```python
from build123d import *

# Parameters (mm, degrees)
F0_R     = 24.686614
F1_DEPTH = 127
F2_R     = 5.08
F3_W     = 13.125889
F3_H     = 11.96772
F4_DEPTH = 127.001


with BuildPart() as f1:
    # F0 (on Front) → F1 (new body)
    with BuildSketch(Plane.XZ):
        with Locations((-110.139199, 36.395181)):
            Circle(F0_R)
    extrude(amount=F1_DEPTH)

    # F2
    f2_edges = [f1.edges().sort_by_distance(p)[0] for p in [
        (-134.825813, -127, 36.395181),
    ]]
    fillet(f2_edges, radius=F2_R)

    # F3 (on face) → F4 (cut, through all)
    with BuildSketch(Plane.XZ.offset(127)):
        with Locations((-109.805476, 36.192703)):
            Rectangle(F3_W, F3_H)
    extrude(amount=-F4_DEPTH, mode=Mode.SUBTRACT)


solid = f1.part
```
Part model, mm, in its own coordinate system. A direction names the side the tool comes from. Round coordinates to 2 decimals unless told otherwise and drop trailing zeros. Order: outer loops, then holes, each group sorted by start corner. A loop starts at its lowest first (then second) coordinate and runs counter-clockwise, first axis right, second up. Notation, with made-up numbers: M 55.5,5.5 L 86.5,5.5 A26 cw 86.5,25.5 Z; hole C 45,82.25 d8. An arc over 180 degrees is marked long. Answer in a Markdown table with one row per item. Add a question column.
Q1. Wall check: L1, parallel to Z at x = -109, y = -11.5; L2, parallel to Y at x = -126.5, z = 25; L3, parallel to Z at x = -116, y = -25. Give the ranges that are in metal, low to high. Write a range as from..to.
Q2. Mould opens along Z. For faces 1 (the face through (-129.73, -60.107, 21.374)), 2 (the face through (-100, 0, 37)), 3 (the face through (-116.368, -64, 36)) say: +Z half, -Z half, draft (parallel to the pull), parting line (faces both ways), or undercut.
Q3. Cut at A-A on y = -72. Give the cut face in (x, z), and give its area (3 significant figures).
Q4. Pin check, flat tips, straight feed: pin 1 (6 mm diameter, centred on x = -129.5, y = -60, fed in from +Z); pin 2 (10.5 mm diameter, centred on x = -112, y = -76, fed in from -Z); pin 3 (8 mm diameter, centred on x = -124, y = -106.5, fed in from +Z). Stop position of each tip, or through.
Q5. 3-axis set-ups, long thin cutter, end or side, ignore diameter. For faces 4 (the face through (-102, -127, 37)), 5 (the face through (-110, -64, 42.177)): which of +Z, -Z, +X, -X, +Y, -Y reach the whole face in a straight line?
Established:
| question | item | result |
|---|---|---|
| 1 | L1 | z = 11.73..30.21, 42.18..61.06 |
| 1 | L2 | y = -126.99..0 |
| 1 | L3 | z = 12.41..30.21, 42.18..60.38 |
| 2 | face 1 | parting line |
| 2 | face 2 | draft |
| 2 | face 3 | undercut |
| 3 | outline | C -110.14,36.4 d49.37; hole M -116.37,30.21 L -103.24,30.21 L -103.24,42.18 L -116.37,42.18 Z |
| 3 | area | 1,760 mm2 |
| 4 | pin 1 | stops at z = 54.88 |
| 4 | pin 2 | stops at z = 11.71 |
| 4 | pin 3 | stops at z = 59.03 |
| 5 | face 4 | +Z, -Z, +X, -X, -Y |
| 5 | face 5 | +Y, -Y |
